Autodesk Inventor part; units mm, degrees
ref_plane "YZ Plane" through (0, 0, 0) normal (1, 0, 0) x (0, 1, 0)
ref_plane "XZ Plane" through (0, 0, 0) normal (0, 1, 0) x (-1, 0, 0)
ref_plane "XY Plane" through (0, 0, 0) normal (0, 0, 1) x (1, 0, 0)
sketch "Sketch1" plane through (0, 0, 0) normal (0, 0, 1) x (1, 0, 0)
  line L0 (0, 0) -> (6.35, 0)
  line L1 (6.35, 0) -> (6.35, -19.05)
  line L2 (6.35, -19.05) -> (0, -19.05)
  line L3 (0, -19.05) -> (0, 0)
  dimension "d0" = 12.7
  dimension "d1" = 19.05
revolve "Revolution1" add sketch "Sketch1" angle 360 about axis through (0, -19.05, 0) along (0, 1, 0)
chamfer "Chamfer1" distance 3.175 angle 45 1 edges at (-6.35, -19.05, 0)
sketch "Sketch2" plane through (0, 0, 0) normal (0, 1, 0) x (1, 0, 0)
  circle A0 centre (0, 0) radius 9.525
  point P0 (0, 0)
  dimension "d6" = 19.05
extrude "Extrusion1" add sketch "Sketch2" along normal blind 6.35
sketch "Sketch3" plane through (0, 6.35, 0) normal (0, 1, 0) x (1, 0, 0)
  line L0 (10.9985, 0) -> (5.4993, -9.525)
  line L1 (5.4993, -9.525) -> (-5.4993, -9.525)
  line L2 (-5.4993, -9.525) -> (-10.9985, 0)
  line L3 (-10.9985, 0) -> (-5.4993, 9.525)
  line L4 (-5.4993, 9.525) -> (5.4993, 9.525)
  line L5 (5.4993, 9.525) -> (10.9985, 0)
  circle A0 centre (0, 0) radius 9.525 construction
  point P0 (0, 0)
  point P1 (0, 0)
extrude "Extrusion2" add sketch "Sketch3" against normal blind 5.969
sketch "Sketch4" plane through (0, 0, 0) normal (0, 0, 1) x (1, 0, 0)
  line L0 (9.2388, 6.35) -> (10.9985, 6.35)
  line L1 (10.9985, 6.35) -> (10.9985, 5.334)
  line L2 (10.9985, 5.334) -> (9.2388, 6.35)
  line L3 (0, -1.5875) -> (0, 9.525)
  line L4 (5.4993, 0) -> (10.9985, 0) construction
  line L5 (5.4993, 6.35) -> (10.9985, 6.35) construction
  line L6 (5.4993, 6.35) -> (5.4993, 0.381) construction
  line L7 (10.9985, 6.35) -> (10.9985, 0.381) construction
  line L8 (10.9985, 6.35) -> (5.4993, 6.35)
  line L9 (8.2489, 0.381) -> (10.9985, 0.381)
  line L10 (5.4993, 0.381) -> (8.2489, 0.381)
  point P0 (0, 0)
  point P1 (16.2522, 7.9375)
  dimension "d11" = 30
  dimension "d17" = 1.016
revolve "Revolution2" cut sketch "Sketch4" angle 360 about axis through (0, -10, 0) along (0, 1, 0)
thread "Thread3"
equation "\"diameter\" = 1.8542"
equation "\"length\" = 19.05"
properties part number "Door Plate Screw" material "Steel, Carbon"
Build history of the part. All positions in model axes, mm. A direction names the side the tool comes from. Give positions to 0.01 mm unless a question says otherwise; leave off trailing zeros. Order: outer loops, then holes, each group sorted by start corner. A loop starts at its lowest first (then second) coordinate and runs counter-clockwise, first axis right, second up. Notation, with made-up numbers: M 35,-10 L 77,-10 A32 ccw 77,27 Z; hole C 80.25,80.25 d8. An arc over 180 degrees is marked long. Put each result on its own line as item: value.
Item 1: Drop flat-ended pins along their axis: pin 1 Ø5 at (x, z) = (1, 7) entering from -Y; pin 2 Ø6 at (y, z) = (-0.5, -7) entering from -X; pin 3 Ø10 at (y, z) = (-11, 6.5) entering from -X. Give the stop position or say it passes through.
Results are:
pin 1: y = -17.65
pin 2: x = -8.62
pin 3: x = -6.17
Item 2: Cut at A-A on y = -14.5. Write the cut outline in (x, z).
Results are:
outline: C 0,0 d12.7
Item 3: Which spindle directions (+Z, -Z, +X, -X, +Y, -Y) get a long thin tool onto all of the face, cutting with end or side? Do faces 1 (the face through (-10, 0.381, -1)), 2 (the face through (-7.559, 0.188, -5.796)), 3 (the face through (10, 0.381, -1)). Say none if no direction does.
Results are:
face 1: -X, -Y
face 2: -Y
face 3: +X, -Y
Item 4: Wall check: probe 1 along Y at (x, z) = (4, -6); probe 2 along X at (y, z) = (-8.75, -5.5); probe 3 along Z at (x, y) = (-2.75, -15). Give the ranges that are in metal, low to high.
Results are:
probe 1: 0 to 6.35
probe 2: -3.17 to 3.17
probe 3: -5.72 to 5.72
